from build123d import *

# Parameters (mm, degrees)
EXTRUDE_1_DEPTH     = 10
HOLE_WIZARD_M6_1_D  = 5
SKETCH_5_W          = 5
SKETCH_5_H          = 0.2
CUT_EXTRUDE_1_DEPTH = 10
EXTRUDE_2_DEPTH     = 2.5
CUT_EXTRUDE_2_DEPTH = 0.3


with BuildPart() as part:
    # 草图1 → 凸台-拉伸1 (new, symmetric)
    with BuildSketch(Plane.XY):
        with BuildLine():
            Line((-0.162539896, 4.7), (-0.162539896, 4.3))
            Line((-0.162539896, 4.3), (-2.412539896, 4.3))
            ThreePointArc((-2.412539896, 4.3), (-2.673218708, 4.148480829), (-2.670578604, 3.846977045))
            Line((-2.670578604, 3.846977045), (-0.251308863, 0.136159055))
            ThreePointArc((-0.251308863, 0.136159055), (-0.142912065, 0.036227102), (0, 0))
            Line((0, 0), (6.374920209, 0))
            ThreePointArc((6.374920209, 0), (6.517832273, 0.036227102), (6.626229072, 0.136159055))
            Line((6.626229072, 0.136159055), (9.045498813, 3.846977045))
            ThreePointArc((9.045498813, 3.846977045), (9.048138917, 4.148480829), (8.787460104, 4.3))
            Line((8.787460104, 4.3), (6.537460104, 4.3))
            Line((6.537460104, 4.3), (6.537460104, 4.7))
            ThreePointArc((6.537460104, 4.7), (6.449592139, 4.912132034), (6.237460104, 5))
            Line((6.237460104, 5), (0.137460104, 5))
            ThreePointArc((0.137460104, 5), (-0.07467193, 4.912132034), (-0.162539896, 4.7))
        make_face()
    extrude(amount=EXTRUDE_1_DEPTH, both=True)

    # M6 螺纹孔1 (through all)
    with Locations(Plane(origin=(3.187460104, 5, 0), x_dir=(1, 0, 0), z_dir=(0, 1, 0))):
        with Locations((0, 0)):
            Hole(HOLE_WIZARD_M6_1_D / 2)

    # 草图5 → 切除-拉伸1 (cut)
    with BuildSketch(Plane.XY.offset(10)):
        with Locations((3.187460104, 0.1)):
            Rectangle(SKETCH_5_W, SKETCH_5_H)
    extrude(amount=-CUT_EXTRUDE_1_DEPTH, mode=Mode.SUBTRACT)

    # 草图6 → 凸台-拉伸2 (add, symmetric)
    with BuildSketch(Plane.ZY.offset(-3.187460104)):
        Polygon((3.00315896, 0.2), (-2.998839756, -2.5), (-3.039864859, -2.408802736), (3.00315896, 0.309652412), align=None)
    extrude(amount=EXTRUDE_2_DEPTH, both=True)

    # 草图7 → 切除-拉伸2 (cut)
    with BuildSketch(Plane(origin=(0, -0.957256199, 0.430621841), x_dir=(1, 0, 0), z_dir=(-1.0372120907131427e-12, -0.9119726400165361, 0.41025102542378794))):
        with BuildLine():
            Line((5.687460104, 0.830780993), (4.156276113, -3.008268608))
            ThreePointArc((4.156276113, -3.008268608), (3.187460104, -3.760487373), (2.218644095, -3.008268608))
            Line((2.218644095, -3.008268608), (0.687460104, 0.830780993))
            Line((0.687460104, 0.830780993), (-4.835906094, -0.220154239))
            Line((-4.835906094, -0.220154239), (4.418162479, -8.671425065))
            Line((4.418162479, -8.671425065), (7.352023336, -1.665190183))
            Line((7.352023336, -1.665190183), (5.687460104, 0.830780993))
        make_face()
    extrude(amount=-CUT_EXTRUDE_2_DEPTH, mode=Mode.SUBTRACT)


solid = part.part
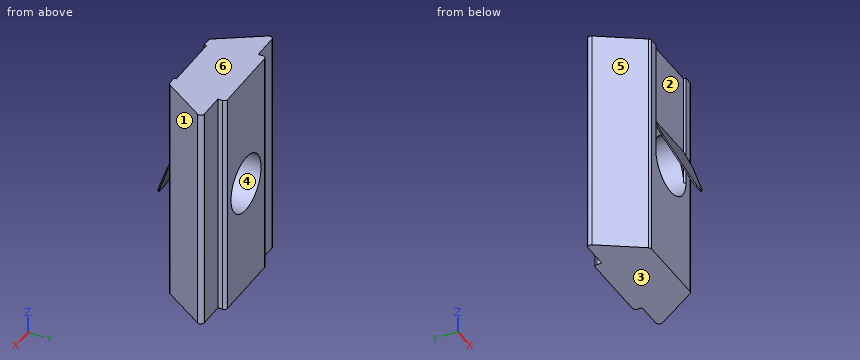
The model under review builds one solid part; all positions refer to its coordinate system, in mm. Face numbers are marked on the shaded views. A direction names the side the tool comes from. Give positions to 0.01 mm unless a question says otherwise; leave off trailing zeros. Order: outer loops, then holes, each group sorted by start corner. A loop starts at its lowest first (then second) coordinate and runs counter-clockwise, first axis right, second up. Notation, with made-up numbers: (-22, -34.5) -> (6, -34.5) arc R5 cw to (6, -28.5) -> close; hole circle Ø10 at (-28, -25). An arc over 180 degrees is marked (long way). Write item = value, one per line. Start each with the question number.
(1) Take a section at D-D (z = -5.5). Write out the cut boundary in (x, y).
(2) Tool access review of the marked faces 1 and 2: name each direction out of +Z, -Z, +X, -X, +Y, -Y from which nothing blocks a thin tool from reaching the whole face with its end or side.
(3) For L1, parallel to Y at x = 1, z = 6.5; L2, parallel to X at y = 2.5, z = -1.75; L3, parallel to Y at x = -0.25, z = -7.75, list the stretches that pass through material, from the lowest coordinate up. Write a range as from..to.
(4) For pin 1 Ø0.7 at (y, z) = (-0.5, 1.5) entering from +X; pin 2 Ø7 at (x, z) = (4.5, 5) entering from -Y; pin 3 Ø4.5 at (x, z) = (3.19, 0) entering from +Y, all flat-tipped, find the tip position at first contact; note any pin that passes through.
(5) Take a section at B-B (x = 1). Write out the cut boundary in (y, z), plus the area to 3 significant figures.
(6) Draft analysis for pull direction Z (two halves, no side actions). For the marked faces 3, 4, 5 and 6, state which applies: +Z half, -Z half, draft (parallel to the pull), parting line (faces both ways), or undercut.
(7) Take a section at C-C (y = 0.75). Write out the cut boundary in (x, z), plus the area to 3 significant figures.
(8) Take a section at A-A (z = -1.5). Write out the cut boundary in (x, y).
Returned:
q1.outline = (-2.67, 3.85) -> (-0.25, 0.14) arc R0.3 ccw to (0, 0) -> (6.37, 0) arc R0.3 ccw to (6.63, 0.14) -> (9.05, 3.85) arc R0.3 ccw to (8.79, 4.3) -> (6.54, 4.3) -> (6.54, 4.7) arc R0.3 ccw to (6.24, 5) -> (0.14, 5) arc R0.3 ccw to (-0.16, 4.7) -> (-0.16, 4.3) -> (-2.41, 4.3) arc R0.3 ccw to start
q2.face_1 = +Z, -Z, +X, -Y
q2.face_2 = +Z, -Y
q3.L1 = 0.2..5
q3.L2 = -1.79..1.4, 4.97..8.17
q3.L3 = 0.13..4.3
q4.pin_1 = 5.69
q4.pin_2 = -0.48
q4.pin_3 = -0.03
q5.outline = (-0.94, 0.47) -> (-0.85, 0.43) -> (0.2, 2.76) -> (0.2, 1.21) -> (5, 1.21) -> (5, 10) -> (0.2, 10) -> (0.2, 3) -> close; (0, -10) -> (5, -10) -> (5, -1.21) -> (0, -1.21) -> close
q5.area = 86.4 mm²
q6.face_3 = -Z half
q6.face_4 = undercut
q6.face_5 = draft
q6.face_6 = +Z half
q7.outline = (-0.65, -10) -> (7.03, -10) -> (7.03, 10) -> (-0.65, 10) -> close; hole circle Ø5 at (3.19, 0)
q7.area = 134 mm²
q8.outline = (-2.67, 3.85) -> (-0.25, 0.14) arc R0.3 ccw to (0, 0) -> (1.19, 0) -> (1.19, 5) -> (0.14, 5) arc R0.3 ccw to (-0.16, 4.7) -> (-0.16, 4.3) -> (-2.41, 4.3) arc R0.3 ccw to start; (1.85, -1.72) -> (1.86, -1.83) -> (4.51, -1.83) -> (4.53, -1.72) -> close; (5.19, 0) -> (6.37, 0) arc R0.3 ccw to (6.63, 0.14) -> (9.05, 3.85) arc R0.3 ccw to (8.79, 4.3) -> (6.54, 4.3) -> (6.54, 4.7) arc R0.3 ccw to (6.24, 5) -> (5.19, 5) -> close
